Source: CAD feature listing. Evaluate the final solid. Frame: model axes, mm. Face numbers are marked on the shaded views. Give positions to 0.01 mm unless a question says otherwise; leave off trailing zeros. Loops run counter-clockwise (first coordinate to the right, second up) from the corner with the lowest first, then second, coordinate; pieces in that order, holes last.
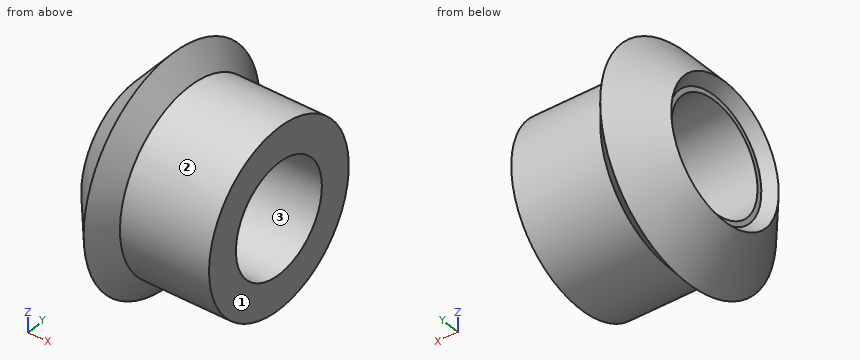
```python
from build123d import *

# Parameters (mm, degrees)
F2_R     = 8
F3_DEPTH = 21.001


with BuildPart() as f1:
    # F0 (on Front) → F1 (revolve)
    with BuildSketch(Plane.XZ):
        Polygon((-142.29493, 2.214532), (-147.655754, -4.174249), (-146.123665, -5.459824), (-146.123665, -14.174249), (-126.655754, -14.174249), (-126.655754, -1.174249), (-139.655754, -1.174249), align=None)
    revolve(axis=Axis((-136.38971, 0, -14.174249), (1, 0, 0)))

    # F2 (on face) → F3 (cut, through all)
    with BuildSketch(Plane.YZ.offset(-126.655754)):
        with Locations((0, -14.174249)):
            Circle(F2_R)
    extrude(amount=-F3_DEPTH, mode=Mode.SUBTRACT)


solid = f1.part
```
(1) Section A-A, the plane y = 0. Return the cut outline in (x, z), then the cut area to 3 significant figures.
A:
outline: (-147.66, -24.17) - (-142.29, -30.56) - (-139.66, -27.17) - (-126.66, -27.17) - (-126.66, -22.17) - (-146.12, -22.17) - (-146.12, -22.89) - close; (-147.66, -4.17) - (-146.12, -5.46) - (-146.12, -6.17) - (-126.66, -6.17) - (-126.66, -1.17) - (-139.66, -1.17) - (-142.29, 2.21) - close
area: 217 mm2
(2) Section C-C, the plane x = -134. Return the cut outline in (y, z), then the cut area to 3 significant figures.
A:
outline: circle Ø26 at (0, -14.17); hole circle Ø16 at (0, -14.17)
area: 330 mm2
(3) First-contact query: pin 1 (2 mm diameter, centred on x = -140, y = -0.5, fed in from -Z); pin 2 (8 mm diameter, centred on x = -129.5, z = -18, fed in from -Y); pin 3 (2 mm diameter, centred on x = -132.5, y = 2, fed in from +Z). Flat tips, straight axial feed; report the tip coordinate or a pass-through.
A:
pin 1: stops at z = -28.89
pin 2: stops at y = -13
pin 3: stops at z = -1.21
(4) Ray query, line 1 along Z through (x, y) = (-137.25, 0); line 2 along Y through (x, z) = (-130, -21.5); line 3 along Y through (x, z) = (-145.5, -17). Return the intervals inside material, ascending.
A:
line 1: z = -27.17 to -22.17, -6.17 to -1.17
line 2: y = -10.74 to -3.21, 3.21 to 10.74
line 3: y = -12.25 to -7.48, 7.48 to 12.25
(5) Section B-B, the plane x = -141.75. Return the cut outline in (y, z), then the cut area to 3 significant figures.
A:
outline: circle Ø31.38 at (0, -14.17); hole circle Ø16 at (0, -14.17)
area: 572 mm2
(6) Mould query, pull axis Y, two halves, no side actions, for the marked faces 1, 2 and 3. Classes: pulls with the +Y half, pulls with the -Y half, needs draft (parallel to the pull), parting line crosses it, or undercut.
A:
face 1: needs draft
face 2: parting line crosses it
face 3: undercut
